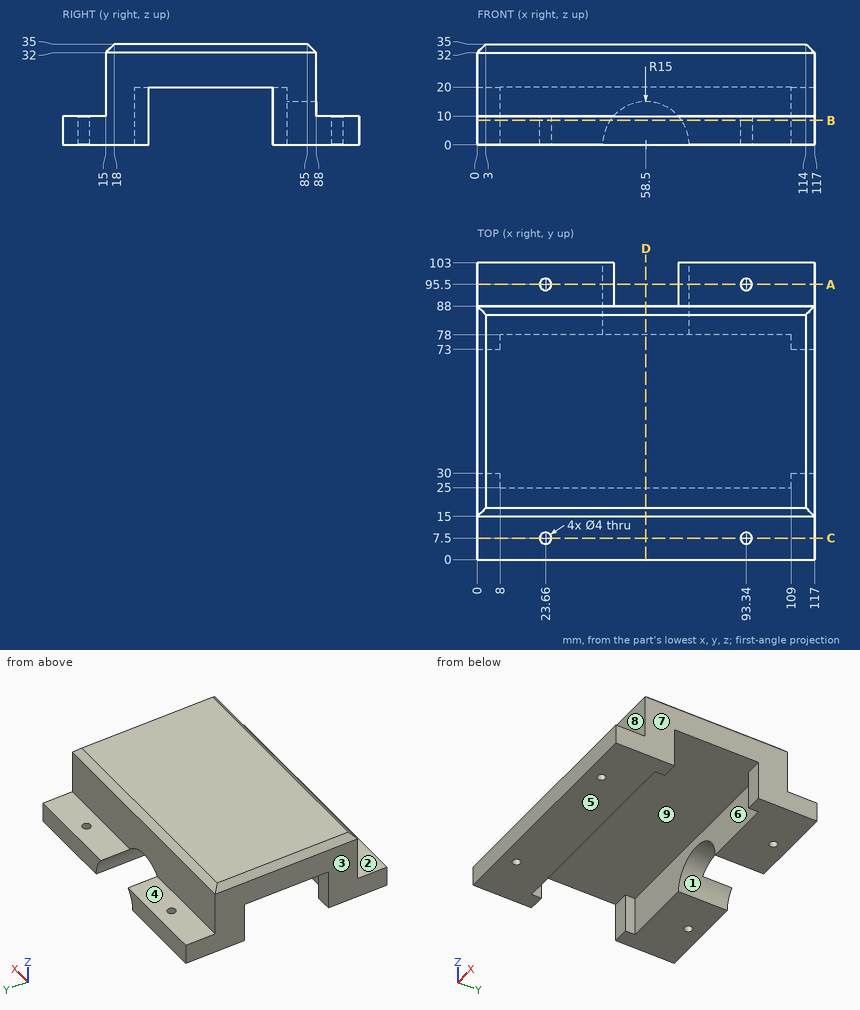
Design review of the part shown in the three views and the two pictorial views. Dimensions are in mm from the part's minimum x, y and z. A direction names the side the tool comes from. Round coordinates to 2 decimals unless told otherwise and drop trailing zeros. Write each loop counter-clockwise with the first axis right and the second up, starting at its lowest first coordinate (ties: lowest second). Pieces come first, ordered by that corner, then holes. Notation, with made-up numbers: (4.5, 72) -> (60.5, 72) arc R26 ccw to (60.5, 103) -> close; hole circle Ø3 at (-28.75, 20.25). An arc over 180 degrees is marked (long way). One line per question, with ' | ' between items. Start each with the question number.
1) Add section B-B (z = 8.5). Write out the cut boundary in (x, y), and give its area (3 significant figures).
2) Add section C-C (y = 7.5). Write out the cut boundary in (x, z).
3) Wall thickness on line 1 along Y through (x, z) = (79, 4); line 2 along Y through (x, z) = (80, 16.5); line 3 along X through (y, z) = (26, 18): over which ranges is each line inside the solid? List them lowest first.
4) Machinability: for the marked faces 1, 2, 3, 4 and 5, which of the approach directions +Z, -Z, +X, -X, +Y, -Y give a long, thin tool a straight path to every point of the face, cutting with its end or side? Answer none if there is none.
5) For pin 1 Ø12 at (x, y) = (18.5, 97) entering from +Z; pin 2 Ø4 at (x, z) = (112.5, 13.5) entering from -Y; pin 3 Ø16 at (x, z) = (63, 12) entering from -Y; pin 4 Ø3.5 at (x, y) = (23.66, 95.5) entering from +Z, all flat-tipped, find the tip position at first contact; note any pin that passes through.
6) Mouldability with a two-part tool opening along Y and no side actions: class the marked faces 6, 7, 8 and 9 as +Y half, -Y half, draft (parallel to the pull), parting line (faces both ways), or undercut.
7) Add section D-D (x = 58.5). Write out the cut boundary in (y, z), and give its area (3 significant figures).
8) Add section A-A (y = 95.5). Write out the cut boundary in (x, z), and give its area (3 significant figures).
Reported:
1) outline: (0, 0) -> (117, 0) -> (117, 30) -> (109, 30) -> (109, 25) -> (8, 25) -> (8, 30) -> (0, 30) -> close; (0, 73) -> (8, 73) -> (8, 78) -> (46.14, 78) -> (46.14, 103) -> (0, 103) -> close; (70.86, 78) -> (109, 78) -> (109, 73) -> (117, 73) -> (117, 103) -> (70.86, 103) -> close; hole circle Ø4 at (23.66, 7.5); hole circle Ø4 at (23.66, 95.5); hole circle Ø4 at (93.34, 7.5); hole circle Ø4 at (93.34, 95.5) | area: 5,340 mm²
2) outline: (0, 0) -> (21.66, 0) -> (21.66, 10) -> (0, 10) -> close; (25.66, 0) -> (91.34, 0) -> (91.34, 10) -> (25.66, 10) -> close; (95.34, 0) -> (117, 0) -> (117, 10) -> (95.34, 10) -> close
3) line 1: y = 0 to 25, 78 to 103 | line 2: y = 15 to 25, 78 to 88 | line 3: x = 0 to 8, 109 to 117
4) face 1: -Z, +Y | face 2: +Z, +X, -X, -Y | face 3: +Z, -Z, -X, +Y, -Y | face 4: +Z, +X, -X, +Y | face 5: -Z, +X, -X, +Y, -Y
5) pin 1: stops at z = 10 | pin 2: stops at y = 15 | pin 3: stops at y = 0 | pin 4: passes through
6) face 6: undercut | face 7: draft | face 8: -Y half | face 9: undercut
7) outline: (0, 0) -> (25, 0) -> (25, 20) -> (78, 20) -> (78, 15) -> (88, 15) -> (88, 32) -> (85, 35) -> (18, 35) -> (15, 32) -> (15, 10) -> (0, 10) -> close | area: 1,490 mm²
8) outline: (0, 0) -> (21.66, 0) -> (21.66, 10) -> (0, 10) -> close; (25.66, 0) -> (43.5, 0) arc R15 cw to (47.32, 10) -> (25.66, 10) -> close; (69.68, 10) arc R15 cw to (73.5, 0) -> (91.34, 0) -> (91.34, 10) -> close; (95.34, 0) -> (117, 0) -> (117, 10) -> (95.34, 10) -> close | area: 814 mm²
